Verification items for the finished model (mm, model axes). A direction names the side the tool comes from. Give positions to 0.01 mm unless a question says otherwise; leave off trailing zeros. Order: outer loops, then holes, each group sorted by start corner. A loop starts at its lowest first (then second) coordinate and runs counter-clockwise, first axis right, second up. Notation, with made-up numbers: (-13, 85.25) - (44, 85.25) arc R18 ccw to (44, 113.25) - close; hole circle Ø2 at (69.25, 60). An arc over 180 degrees is marked (long way). Answer as a JSON object with one key per item and string values. Group by question number.
(1) Depth check by flat-ended pin: pin 1 Ø10 at (x, z) = (11.5, 2.5) entering from +Y; pin 2 Ø10 at (y, z) = (6.5, -1.5) entering from -X; pin 3 Ø2.5 at (x, y) = (0, 5.3) entering from +Z; pin 4 Ø5 at (x, y) = (0, 5.3) entering from -Z. Enter the tip coordinate at first touch or a pass-through.
(2) Section check C-C (y = 5.3). Record the boundary of the cut face in (x, z).
(3) Thickness scan on line 1 (Z direction, x = 0, y = 8); line 2 (X direction, y = 39, z = 8); line 3 (Y direction, x = 3.75, z = -7). Record the ranges inside material, lowest first.
(4) Mould release check, pull along X, two halves, no side actions. Record for faces 1 (the face through (-6, 15.8, 0)), 2 (the face through (1.432, 4.706, 3.537)), 3 (the face through (-1.72, 7.05, 4.16)): +X half, -X half, draft (parallel to the pull), parting line (faces both ways), or undercut.
(5) Section check A-A (x = 0). Record the boundary of the cut face in (y, z), then the cut area to 3 significant figures.
(6) Section check B-B (z = 0). Record the boundary of the cut face in (x, y), then the cut area to 3 significant figures.
(7) Access from +Z, -Z, +X, -X, +Y, -Y to the whole of each face (thin tool, end or side, straight path). Record for faces 4 (the face through (5.8, 28, 0)), 5 (the face through (-4, 14.3, -3)), 6 (the face through (3.8, 28, 0)).
(8) Section check D-D (z = 10.75). Record the boundary of the cut face in (x, y), then the cut area to 3 significant figures.
```python
from build123d import *

# Parameters (mm, degrees)
SKETCH_1_R               = 4.5
SKETCH_1_R_2             = 3.1
EXTRUDE_1_DEPTH          = 14.3
EXTRUDE_START            = -11.25
EXTRUDE_2_DEPTH          = 11.25
CUT_EXTRUDE_1_DEPTH      = 16.652156401
CUT_EXTRUDE_1_DEPTH_BACK = 16.652156401
SKETCH_3_R               = 1.55
SKETCH_4_W               = 30
SKETCH_4_H               = 25
EXTRUDE_3_DEPTH          = 1.5
SKETCH_5_R               = 1.6
CUT_EXTRUDE_2_DEPTH      = 26.117523826
SKETCH_6_W               = 2
SKETCH_6_H               = 25
EXTRUDE_4_DEPTH          = 25


with BuildPart() as part:
    # 草图1 → 凸台-拉伸1 (new body)
    with BuildSketch(Plane(origin=(0, 0, 0), x_dir=(1, 0, 0), z_dir=(0, 1, 0))):
        with Locations(Location((0, 0, 0), (0, 0, 270))):
            Circle(SKETCH_1_R)
        with Locations(Location((0, 0, 0), (0, 0, 270))):
            Circle(SKETCH_1_R_2, mode=Mode.SUBTRACT)
    extrude(amount=EXTRUDE_1_DEPTH)

    # 草图2 → 凸台-拉伸2 (add)
    with BuildSketch(Plane(origin=(0, 14.3, 0), x_dir=(1, 0, 0), z_dir=(0, 1, 0)).offset(EXTRUDE_START)):
        with BuildLine():
            Line((-1.688194302, -2.6), (1.688194302, -2.6))
            ThreePointArc((1.688194302, -2.6), (0, -3.1), (-1.688194302, -2.6))
        make_face()
    extrude(amount=EXTRUDE_2_DEPTH)

    # 草图3 → 切除-拉伸1 (cut, two sides: drawn at the far end of the back side and taken through both)
    with BuildSketch(Plane.XY.offset(-CUT_EXTRUDE_1_DEPTH_BACK)):
        with Locations((0, 5.3)):
            Circle(SKETCH_3_R)
    extrude(amount=CUT_EXTRUDE_1_DEPTH + CUT_EXTRUDE_1_DEPTH_BACK, mode=Mode.SUBTRACT)

    # 草图4 → 凸台-拉伸3 (add)
    with BuildSketch(Plane(origin=(0, 14.3, 0), x_dir=(1, 0, 0), z_dir=(0, 1, 0))):
        Rectangle(SKETCH_4_W, SKETCH_4_H)
    extrude(amount=EXTRUDE_3_DEPTH)

    # 草图5 → 切除-拉伸2 (cut, through all)
    with BuildSketch(Plane(origin=(0, 15.8, 0), x_dir=(1, 0, 0), z_dir=(0, 1, 0))):
        with Locations(Location((0, 0, 0), (0, 0, 270))):
            Circle(SKETCH_5_R)
    extrude(amount=-CUT_EXTRUDE_2_DEPTH, mode=Mode.SUBTRACT)

    # 草图6 → 凸台-拉伸4 (add)
    with BuildSketch(Plane(origin=(0, 15.8, 0), x_dir=(1, 0, 0), z_dir=(0, 1, 0))):
        with Locations((4.8, 0)):
            Rectangle(SKETCH_6_W, SKETCH_6_H)
    extrude(amount=EXTRUDE_4_DEPTH)


solid = part.part
```
Solutions:
{
 "1": {"pin 1": "stops at y = 15.8", "pin 2": "stops at x = -4.5", "pin 3": "passes through", "pin 4": "stops at z = -4.5"},
 "2": {"outline": "(-1.69, 2.6) - (-1.55, 2.6) - (-1.55, 4.22) arc R4.5 ccw to (-1.55, -4.22) - (-1.55, -2.68) arc R3.1 cw to start; (1.55, -4.22) arc R4.5 ccw to (1.55, 4.22) - (1.55, 2.6) - (1.69, 2.6) arc R3.1 cw to (1.55, -2.68) - close"},
 "3": {"line 1": "z = -4.5 to -3.1, 2.6 to 4.5", "line 2": "x = 3.8 to 5.8", "line 3": "y = 14.3 to 15.8"},
 "4": {"face 1": "draft", "face 2": "undercut", "face 3": "parting line"},
 "5": {"outline": "(0, -4.5) - (3.75, -4.5) - (3.75, -3.1) - (0, -3.1) - close; (0, 3.1) - (3.05, 3.1) - (3.05, 2.6) - (3.75, 2.6) - (3.75, 4.5) - (0, 4.5) - close; (6.85, -4.5) - (14.3, -4.5) - (14.3, -12.5) - (15.8, -12.5) - (15.8, -1.6) - (14.3, -1.6) - (14.3, -3.1) - (6.85, -3.1) - close; (6.85, 2.6) - (14.3, 2.6) - (14.3, 1.6) - (15.8, 1.6) - (15.8, 12.5) - (14.3, 12.5) - (14.3, 4.5) - (6.85, 4.5) - close", "area": "68.1 mm2"},
 "6": {"outline": "(-15, 14.3) - (-4.5, 14.3) - (-4.5, 0) - (-3.1, 0) - (-3.1, 14.3) - (-1.6, 14.3) - (-1.6, 15.8) - (-15, 15.8) - close; (1.6, 14.3) - (3.1, 14.3) - (3.1, 0) - (4.5, 0) - (4.5, 14.3) - (15, 14.3) - (15, 15.8) - (5.8, 15.8) - (5.8, 40.8) - (3.8, 40.8) - (3.8, 15.8) - (1.6, 15.8) - close", "area": "130 mm2"},
 "7": {"face 4": "+Z, -Z, +X, +Y", "face 5": "-Y", "face 6": "+Z, -Z, -X, +Y"},
 "8": {"outline": "(-15, 14.3) - (15, 14.3) - (15, 15.8) - (5.8, 15.8) - (5.8, 40.8) - (3.8, 40.8) - (3.8, 15.8) - (-15, 15.8) - close", "area": "95.0 mm2"}
}
